```python
from build123d import *

# Parameters (mm, degrees)
SKETCH3_R           = 14
SKETCH3_R_2         = 5
BOSS_EXTRUDE1_DEPTH = 5
SKETCH4_R           = 1.5
CUT_EXTRUDE1_DEPTH  = 1
SKETCH5_R           = 1.5
CUT_EXTRUDE2_DEPTH  = 1
SKETCH6_R           = 1
CUT_EXTRUDE3_DEPTH  = 30


with BuildPart() as part:
    # Sketch3 → Boss-Extrude1 (new body)
    with BuildSketch(Plane.XY):
        Circle(SKETCH3_R)
        Circle(SKETCH3_R_2, mode=Mode.SUBTRACT)
    extrude(amount=BOSS_EXTRUDE1_DEPTH)

    # Sketch4 → Cut-Extrude1 (cut)
    with BuildSketch(Plane.XY.offset(5)):
        with Locations((0, 11)):
            Circle(SKETCH4_R)
        with Locations((9.526279442, -5.5)):
            Circle(SKETCH4_R)
        with Locations((-9.526279442, -5.5)):
            Circle(SKETCH4_R)
    extrude(amount=-CUT_EXTRUDE1_DEPTH, mode=Mode.SUBTRACT)

    # Sketch5 → Cut-Extrude2 (cut)
    with BuildSketch(Plane(origin=(0, 0, 0), x_dir=(-1, 0, 0), z_dir=(0, 0, -1))):
        with Locations((0, 11)):
            Circle(SKETCH5_R)
        with Locations((9.526279442, -5.5)):
            Circle(SKETCH5_R)
        with Locations((-9.526279442, -5.5)):
            Circle(SKETCH5_R)
    extrude(amount=-CUT_EXTRUDE2_DEPTH, mode=Mode.SUBTRACT)

    # Sketch6 → Cut-Extrude3 (cut)
    with BuildSketch(Plane(origin=(0, 0, 0), x_dir=(1, 0, 0), z_dir=(0, 1, 0))):
        with Locations((0, -2.5)):
            Circle(SKETCH6_R)
    extrude(amount=-CUT_EXTRUDE3_DEPTH, mode=Mode.SUBTRACT)


solid = part.part
```
The model under review builds one solid part; all positions refer to its coordinate system, in mm. A direction names the side the tool comes from. Round coordinates to 2 decimals unless told otherwise and drop trailing zeros. Loops run counter-clockwise (first coordinate to the right, second up) from the corner with the lowest first, then second, coordinate; pieces in that order, holes last. Notation, with made-up numbers: (-34, -39.75) - (-8, -39.75) arc R9 ccw to (-8, -25.75) - close; hole circle Ø1 at (5, -37.75). An arc over 180 degrees is marked (long way). Write each question's results on one line, items separated by ' | '. Start each with the question number.
Q1. Take a section at B-B on y = 0. Give the boundary of the cut face in (x, z).
Q2. Wall thickness on line 1 along Y through (x, z) = (0, 4.7); line 2 along X through (y, z) = (-6.25, 4.3); line 3 along Z through (x, y) = (0, -11.75): over which ranges is each line inside the solid? List them lowest first. Write a range as [from, to].
Q3. Tool access review of faces 1 (the cylindrical face through (-0.217, -9.386, 3.476)), 2 (the cylindrical face through (2.307, -4.436, 2.465)), 3 (the flat face through (0, 11, 4)), 4 (the flat face through (6, 0, 5)), 5 (the cylindrical face through (0.325, 9.536, 0.493)): name each direction out of +Z, -Z, +X, -X, +Y, -Y from which nothing blocks a thin tool from reaching the whole face with its end or side.
Q4. Draft analysis for pull direction Y (two halves, no side actions). For faces 6 (the flat face through (6, 0, 0)), 7 (the flat face through (-10, -5, 1)), 8 (the cylindrical face through (12.932, -5.362, 2.465)), state which applies: pulls with the +Y half, pulls with the -Y half, needs draft (parallel to the pull), parting line crosses it, or undercut.
Q5. Take a section at C-C on x = -3. Give the boundary of the cut face in (y, z), plus the area to 3 significant figures.
Q6. Take a section at D-D on y = -5.5. Give the boundary of the cut face in (x, z).
Q7. Take a section at A-A on x = 0. Give the boundary of the cut face in (y, z).
Q8. Insertion check: P1, Ø2.5, axis at x = 0.5, y = 10.5, coming from the +Z side; P2, Ø2.5, axis at x = -9.53, y = -5.5, coming from the +Z side; P3, Ø1.5, axis at x = -0.5, y = 11.5, coming from the -Z side; P4, Ø1.2, axis at x = 0, z = 2.5, coming from the -Y side. Each pin has a flat end and moves straight along its axis. Give the tip position at first contact, or say it passes through.
Data:
1) outline: (-14, 0) - (-5, 0) - (-5, 5) - (-14, 5) - close; (5, 0) - (14, 0) - (14, 5) - (5, 5) - close
2) line 1: y = [-14, -5], [5, 9.5], [12.5, 14] | line 2: x = [-12.53, -10.83], [-8.23, 8.23], [10.83, 12.53] | line 3: z = [0, 1.5], [3.5, 5]
3) face 1: -Y | face 2: +Z, -Z | face 3: +Z | face 4: +Z, +X, -X, +Y, -Y | face 5: -Z
4) face 6: needs draft | face 7: undercut | face 8: parting line crosses it
5) outline: (-13.67, 0) - (-4, 0) - (-4, 5) - (-13.67, 5) - close; (4, 0) - (13.67, 0) - (13.67, 5) - (4, 5) - close | area: 96.7 mm²
6) outline: (-12.87, 0) - (-11.03, 0) - (-11.03, 1) - (-8.03, 1) - (-8.03, 0) - (8.03, 0) - (8.03, 1) - (11.03, 1) - (11.03, 0) - (12.87, 0) - (12.87, 5) - (11.03, 5) - (11.03, 4) - (8.03, 4) - (8.03, 5) - (-8.03, 5) - (-8.03, 4) - (-11.03, 4) - (-11.03, 5) - (-12.87, 5) - close; hole circle Ø2 at (0, 2.5)
7) outline: (-14, 0) - (-5, 0) - (-5, 1.5) - (-14, 1.5) - close; (-14, 3.5) - (-5, 3.5) - (-5, 5) - (-14, 5) - close; (5, 0) - (9.5, 0) - (9.5, 1) - (12.5, 1) - (12.5, 0) - (14, 0) - (14, 5) - (12.5, 5) - (12.5, 4) - (9.5, 4) - (9.5, 5) - (5, 5) - close
8) P1: stops at z = 5 | P2: stops at z = 4 | P3: stops at z = 1 | P4: stops at y = 4.96
